Design review of the part shown in the three views and the two pictorial views. Dimensions are in mm from the part's minimum x, y and z. Give positions to 0.01 mm unless a question says otherwise; leave off trailing zeros. Loops run counter-clockwise (first coordinate to the right, second up) from the corner with the lowest first, then second, coordinate; pieces in that order, holes last. Notation, with made-up numbers: (28.5, -12.75) - (70.5, -12.75) arc R18 ccw to (70.5, -8.75) - close; hole circle Ø8 at (18, 56). An arc over 180 degrees is marked (long way). Answer as a JSON object with one key per item and string values.
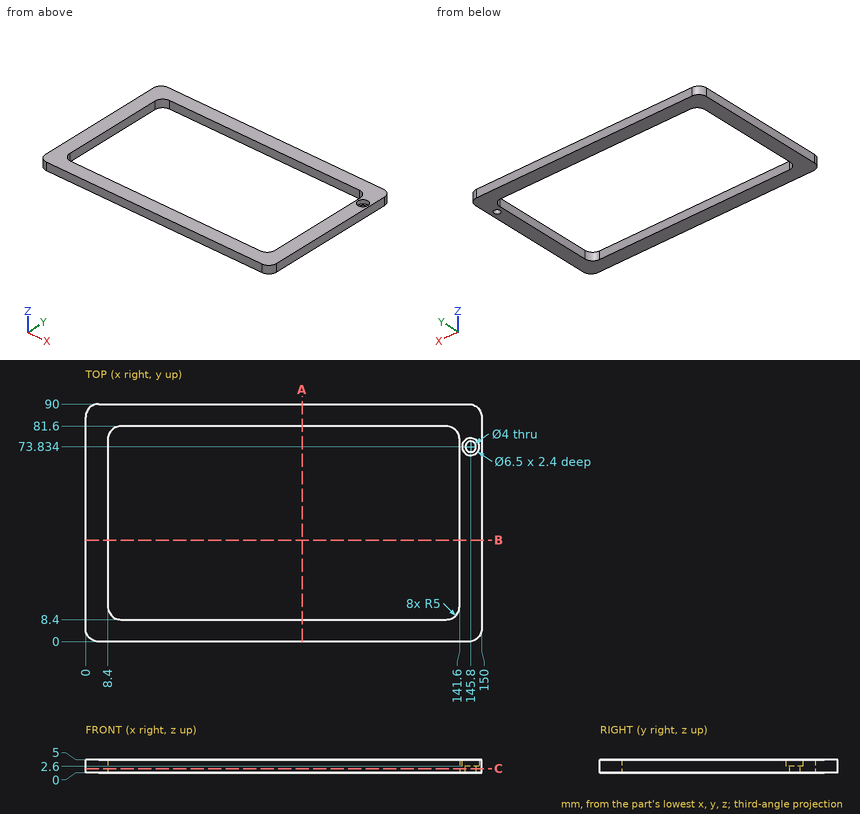
Q1. Consider section A-A, the plane x = 82. State the section outline as (y, z) points.
Results:
{"outline": "(0, 0) - (8.4, 0) - (8.4, 5) - (0, 5) - close; (81.6, 0) - (90, 0) - (90, 5) - (81.6, 5) - close"}
Q2. To check wall thickness, follow probe 1 along X at (y, z) = (54, 0.8); probe 2 along Y at (x, z) = (20, 2.15); probe 3 along X at (y, z) = (74.5, 3.8). State the ranges of each line that lie inside material, in increasing order. Write a range as [from, to].
Results:
{"probe 1": "x = [0, 8.4], [141.6, 150]", "probe 2": "y = [0, 8.4], [81.6, 90]", "probe 3": "x = [0, 8.4], [141.6, 142.62], [148.98, 150]"}
Q3. Consider section B-B, the plane y = 38.5. State the section outline as (x, z) points.
Results:
{"outline": "(0, 0) - (8.4, 0) - (8.4, 5) - (0, 5) - close; (141.6, 0) - (150, 0) - (150, 5) - (141.6, 5) - close"}
Q4. Consider section C-C, the plane z = 1.6. State the section outline as (x, y) points.
Results:
{"outline": "(0, 5) arc R5 ccw to (5, 0) - (145, 0) arc R5 ccw to (150, 5) - (150, 85) arc R5 ccw to (145, 90) - (5, 90) arc R5 ccw to (0, 85) - close; hole (8.4, 13.4) arc R5 ccw to (13.4, 8.4) - (136.6, 8.4) arc R5 ccw to (141.6, 13.4) - (141.6, 76.6) arc R5 ccw to (136.6, 81.6) - (13.4, 81.6) arc R5 ccw to (8.4, 76.6) - close; hole circle Ø4 at (145.8, 73.83)"}
Q5. Clearance check with flat-ended pins moving along their axes: pin 1 Ø7.5 at (x, y) = (145.8, 73.83) entering from -Z; pin 2 Ø4.5 at (x, y) = (145.8, 73.83) entering from +Z. State where each tip first meets the part, or that it passes through.
Results:
{"pin 1": "stops at z = 0", "pin 2": "stops at z = 2.6"}
